```python
from build123d import *

# Parameters (mm, degrees)
SKETCH1_W           = 32.5
SKETCH1_H           = 46.5
BOSS_EXTRUDE2_DEPTH = 10.261196577
SHELL1_T            = -2
CUT_EXTRUDE1_DEPTH  = 6
SKETCH3_R           = 1.5
BOSS_EXTRUDE3_DEPTH = 10.261197
CUT_EXTRUDE2_DEPTH  = 6.5
SKETCH5_W           = 28.5
SKETCH5_H           = 1
CUT_EXTRUDE3_DEPTH  = 6.5
CUT_EXTRUDE4_DEPTH  = 6.5
CUT_EXTRUDE5_DEPTH  = 6
SKETCH9_W           = 20.936862588
SKETCH9_H           = 0.25
CUT_EXTRUDE6_DEPTH  = 6
FILLET1_R           = 0.6


with BuildPart() as part:
    # Sketch1 → Boss-Extrude2 (new body)
    with BuildSketch(Plane(origin=(0, 0, 0), x_dir=(0, 0, -1), z_dir=(1, 0, 0))):
        with Locations((1.653195489, 2.097744361)):
            Rectangle(SKETCH1_W, SKETCH1_H)
    extrude(amount=BOSS_EXTRUDE2_DEPTH)

    # Shell1
    shell1_openings = [part.faces().sort_by_distance(p)[0] for p in [
        (10.261196577, 2.097744361, -1.653195489),
    ]]
    offset(amount=SHELL1_T, openings=shell1_openings, kind=Kind.INTERSECTION)

    # Sketch2 → Cut-Extrude1 (cut)
    with BuildSketch(Plane.ZY):
        with BuildLine():
            Line((5.438656476, 5.910225306), (-8.88311082, -14.580918672))
            ThreePointArc((-8.88311082, -14.580918672), (-8.670273984, -15.781926533), (-7.469266123, -15.569089697))
            Line((-7.469266123, -15.569089697), (6.852501173, 4.922054281))
            ThreePointArc((6.852501173, 4.922054281), (6.639664337, 6.123062142), (5.438656476, 5.910225306))
        make_face()
        with BuildLine():
            Line((9.762292675, -0.098981343), (-1.695121162, -16.491896525))
            ThreePointArc((-1.695121162, -16.491896525), (-1.482506801, -17.689391949), (-0.285011378, -17.476777587))
            Line((-0.285011378, -17.476777587), (11.17208338, -1.084318933))
            ThreePointArc((11.17208338, -1.084318933), (10.959856822, 0.113245215), (9.762292675, -0.098981343))
        make_face()
        with BuildLine():
            Line((2.323350937, 20.471761321), (-11.998416359, -0.019382657))
            ThreePointArc((-11.998416359, -0.019382657), (-11.785579523, -1.220390518), (-10.584571661, -1.007553682))
            Line((-10.584571661, -1.007553682), (3.737195635, 19.483590296))
            ThreePointArc((3.737195635, 19.483590296), (3.524358799, 20.684598157), (2.323350937, 20.471761321))
        make_face()
        with BuildLine():
            Line((-3.125347413, 20.917445103), (-14.581484934, 4.526356034))
            ThreePointArc((-14.581484934, 4.526356034), (-14.368482992, 3.328930591), (-13.171057549, 3.541932534))
            Line((-13.171057549, 3.541932534), (-1.715558185, 19.932108547))
            ThreePointArc((-1.715558185, 19.932108547), (-1.927784521, 21.129671439), (-3.125347413, 20.917445103))
        make_face()
    extrude(amount=-CUT_EXTRUDE1_DEPTH, mode=Mode.SUBTRACT)

    # Sketch3 → Boss-Extrude3 (add)
    with BuildSketch(Plane(origin=(10.261196577, 0, 0), x_dir=(0, 0, -1), z_dir=(1, 0, 0))):
        with Locations((15.903195489, 23.347744361)):
            Circle(SKETCH3_R)
        with Locations((-12.596804511, -19.152255639)):
            Circle(SKETCH3_R)
    extrude(amount=-BOSS_EXTRUDE3_DEPTH)

    # Sketch4 → Cut-Extrude2 (cut)
    with BuildSketch(Plane(origin=(10.261196577, 0, 0), x_dir=(0, 0, -1), z_dir=(1, 0, 0))):
        Polygon((-13.572559932, 24.347744361), (-13.572559932, -20.152255639), (-12.596804511, -20.152255639), (-12.596804511, 23.347744361), (15.903195489, 23.347744361), (15.903195489, -20.152255639), (16.903195489, -20.152255639), (16.903195489, 24.347744361), align=None)
    extrude(amount=-CUT_EXTRUDE2_DEPTH, mode=Mode.SUBTRACT)

    # Sketch5 → Cut-Extrude3 (cut)
    with BuildSketch(Plane(origin=(10.261196577, 0, 0), x_dir=(0, 0, -1), z_dir=(1, 0, 0))):
        with Locations((1.653195489, -19.652255639)):
            Rectangle(SKETCH5_W, SKETCH5_H)
    extrude(amount=-CUT_EXTRUDE3_DEPTH, mode=Mode.SUBTRACT)

    # Sketch6 → Cut-Extrude4 (cut)
    with BuildSketch(Plane(origin=(10.261196577, 0, 0), x_dir=(0, 0, -1), z_dir=(1, 0, 0))):
        with BuildLine():
            Line((-12.596804511, -17.652255639), (-12.596804511, -19.152255639))
            Line((-12.596804511, -19.152255639), (-11.096804511, -19.152255639))
            ThreePointArc((-11.096804511, -19.152255639), (-11.536144339, -18.091595467), (-12.596804511, -17.652255639))
        make_face()
        with BuildLine():
            Line((15.903195489, 23.347744361), (15.903195489, 21.847744361))
            ThreePointArc((15.903195489, 21.847744361), (14.842535317, 22.287084189), (14.403195489, 23.347744361))
            Line((14.403195489, 23.347744361), (15.903195489, 23.347744361))
        make_face()
    extrude(amount=-CUT_EXTRUDE4_DEPTH, mode=Mode.SUBTRACT)

    # Sketch8 → Cut-Extrude5 (cut)
    with BuildSketch(Plane(origin=(10.261196577, 0, 0), x_dir=(0, 0, -1), z_dir=(1, 0, 0))):
        Polygon((17.153195489, 24.304666322), (17.153195489, -20.402255639), (7.364302656, -20.402255639), (7.364302656, -20.152255639), (16.903195489, -20.152255639), (16.903195489, 24.347744361), (-13.572559932, 24.347744361), (-13.572559932, -20.402255639), (-13.822559932, -20.402255639), (-13.822559932, 19.230791598), (-13.822559932, 24.597744361), (15.426743448, 24.597744361), (17.153195489, 24.597744361), align=None)
    extrude(amount=-CUT_EXTRUDE5_DEPTH, mode=Mode.SUBTRACT)

    # Sketch9 → Cut-Extrude6 (cut)
    with BuildSketch(Plane(origin=(10.261196577, 0, 0), x_dir=(0, 0, -1), z_dir=(1, 0, 0))):
        with Locations((-3.104128638, -20.277255639)):
            Rectangle(SKETCH9_W, SKETCH9_H)
    extrude(amount=-CUT_EXTRUDE6_DEPTH, mode=Mode.SUBTRACT)

    # Fillet1
    fillet1_edges = [part.edges().sort_by_distance(p)[0] for p in [
        (7.261196577, 24.597744361, -17.153195489),
        (7.261196577, -20.402255639, -17.153195489),
        (7.261196577, -20.402255639, 13.822559932),
        (7.261196577, 24.597744361, 13.822559932),
    ]]
    fillet(fillet1_edges, radius=FILLET1_R)


solid = part.part
```
Design review of the part built by this model. Coordinates are the model's own, in mm. A direction names the side the tool comes from. Give positions to 0.01 mm unless a question says otherwise; leave off trailing zeros. Write each loop counter-clockwise with the first axis right and the second up, starting at its lowest first coordinate (ties: lowest second). Pieces come first, ordered by that corner, then holes. Notation, with made-up numbers: (42, 50.25) -> (56, 50.25) arc R23 cw to (56, 73.25) -> close; hole circle Ø6 at (-1.5, 55.25). An arc over 180 degrees is marked (long way). Answer in a Markdown table with one row per item.
(1) Consider section C-C (z = 0.5). State the section outline as (x, y) points.
Results:
| item | result |
|---|---|
| outline | (0, -21.15) -> (10.26, -21.15) -> (10.26, -20.4) -> (4.26, -20.4) -> (4.26, -20.15) -> (3.76, -20.15) -> (3.76, -19.15) -> (2, -19.15) -> (2, -16.35) -> (0, -16.35) -> close; (0, -13.35) -> (2, -13.35) -> (2, -4.17) -> (0, -4.17) -> close; (0, -1.16) -> (2, -1.16) -> (2, 14.85) -> (0, 14.85) -> close; (0, 17.86) -> (2, 17.86) -> (2, 23.35) -> (3.76, 23.35) -> (3.76, 24.35) -> (4.26, 24.35) -> (4.26, 24.6) -> (10.26, 24.6) -> (10.26, 25.35) -> (0, 25.35) -> close |
(2) For faces 1 (the flat face through (1, 12.8, -8.8)), 2 (the flat face through (5, -21.152, -1)), 3 (the cylindrical face through (2.893, -18.103, 11.525)), list the 3-axis set-ups (+Z, -Z, +X, -X, +Y, -Y) from which the entire face can be reached by the end or side of a thin tool; tool diameter is ignored.
Results:
| item | result |
|---|---|
| face 1 | +X, -X |
| face 2 | +Z, -Z, +X, -X, -Y |
| face 3 | +X |
(3) Mouldability with a two-part tool opening along Z and no side actions: class faces 4 (the flat face through (3.761, 2, 13)), 5 (the flat face through (0.99, -5.47, -0.41)), 6 (the flat face through (5, 25.348, -1)) as +Z half, -Z half, draft (parallel to the pull), parting line (faces both ways), or undercut.
Results:
| item | result |
|---|---|
| face 4 | undercut |
| face 5 | undercut |
| face 6 | draft |
(4) Clearance check with flat-ended pins moving along their axes: pin 1 (10 mm diameter, centred on y = 18.5, z = 8, fed in from -X); pin 2 (2 mm diameter, centred on y = 8.5, z = 7, fed in from +X). State where each tip first meets the part, or that it passes through.
Results:
| item | result |
|---|---|
| pin 1 | x = 0 |
| pin 2 | x = 2 |
(5) Consider section B-B (y = 2). State the section outline as (x, z) points, then the cut area to 3 significant figures.
Results:
| item | result |
|---|---|
| outline | (0, -17.9) -> (10.26, -17.9) -> (10.26, -17.15) -> (4.26, -17.15) -> (4.26, -16.9) -> (3.76, -16.9) -> (3.76, -15.9) -> (2, -15.9) -> (2, -10.59) -> (0, -10.59) -> close; (0, -8.48) -> (2, -8.48) -> (2, 2.71) -> (0, 2.71) -> close; (0, 4.81) -> (2, 4.81) -> (2, 12.6) -> (3.76, 12.6) -> (3.76, 13.57) -> (4.26, 13.57) -> (4.26, 13.82) -> (10.26, 13.82) -> (10.26, 14.6) -> (0, 14.6) -> close |
| area | 73.8 mm2 |
(6) Consider section D-D (z = 6). State the section outline as (x, y) points, then the cut area to 3 significant figures.
Results:
| item | result |
|---|---|
| outline | (0, -21.15) -> (10.26, -21.15) -> (10.26, -20.4) -> (4.26, -20.4) -> (4.26, -20.15) -> (3.76, -20.15) -> (3.76, -19.15) -> (2, -19.15) -> (2, -8.48) -> (0, -8.48) -> close; (0, -5.48) -> (2, -5.48) -> (2, 3.7) -> (0, 3.7) -> close; (0, 6.27) -> (2, 6.27) -> (2, 23.35) -> (3.76, 23.35) -> (3.76, 24.35) -> (4.26, 24.35) -> (4.26, 24.6) -> (10.26, 24.6) -> (10.26, 25.35) -> (0, 25.35) -> close |
| area | 98.9 mm2 |
(7) To check wall thickness, follow probe 1 along Y at (x, z) = (8.5, 6.5); probe 2 along Z at (x, y) = (5, 19); probe 3 along Z at (x, y) = (2.5, -7.5). State the ranges of each line that lie inside material, in increasing order.
Results:
| item | result |
|---|---|
| probe 1 | -21.15 to -20.4, 24.6 to 25.35 |
| probe 2 | -17.9 to -17.15, 13.82 to 14.6 |
| probe 3 | -17.9 to -15.9, 12.6 to 14.6 |
(8) Consider section A-A (x = 2.5). State the section outline as (y, z) points.
Results:
| item | result |
|---|---|
| outline | (-21.15, -17.9) -> (25.35, -17.9) -> (25.35, 14.6) -> (-21.15, 14.6) -> close; hole (-19.15, -15.9) -> (21.85, -15.9) arc R1.5 cw to (23.35, -14.4) -> (23.35, 12.6) -> (-17.65, 12.6) arc R1.5 cw to (-19.15, 11.1) -> close |
